The listing builds one solid part. Answer for the finished solid, in the listing's coordinates (mm). A direction names the side the tool comes from. Give positions to 0.01 mm unless a question says otherwise; leave off trailing zeros. Write each loop counter-clockwise with the first axis right and the second up, starting at its lowest first coordinate (ties: lowest second). Pieces come first, ordered by that corner, then holes. Notation, with made-up numbers: (-23, -7.75) - (0, -7.75) arc R21 cw to (0, -1.75) - close; hole circle Ø1 at (59.5, 39.25). An arc over 180 degrees is marked (long way). Answer as CSV lines item,"result". Start each with the question number.
(1) For faces 4 (the face through (184.08, -0.99, 126.32)), 5 (the face through (182.017, -1.479, 125.126)), determine the directions among +Z, -Z, +X, -X, +Y, -Y from which every point of the face is accessible in a straight line to the end or side of a thin tool.
(2) Find section A-A (x = 184.15). Write down the section's boundary in (y, z), then the cut area to 3 significant figures.
(3) Find section B-B (y = -0.75). Write down the section's boundary in (x, z), then the cut area to 3 significant figures.
(4) For a pull along X with two mould halves and no side action, classify faces 1 (the face through (183.37, -6.85, 124.21)), 2 (the face through (183.464, -1, 125)), 3 (the face through (183, -3, 126)) as pulls with the +X half, pulls with the -X half, needs draft (parallel to the pull), parting line crosses it, or undercut.
(5) Straight lines are drawn through the part: probe 1 along Y at (x, z) = (182.45, 125.45); probe 2 along Y at (x, z) = (183.5, 125.2); probe 3 along X at (y, z) = (-9, 125.35). For each, find the intervals that lie inside material, in ascending order.
(6) Find section C-C (z = 124.4). Write down the section's boundary in (x, y), then the cut area to 3 significant figures.
(7) Each of these flat-tipped pins is pushed along its axis until it touches: pin 1 Ø2 at (y, z) = (-5, 124) entering from -X; pin 2 Ø1 at (x, z) = (183, 127) entering from -Y. Where does it stop, or does it pass through?
(8) Find section D-D (y = -9.25). Write down the section's boundary in (x, z), then the cut area to 3 significant figures.
from build123d import *

# Parameters (mm, degrees)
SKETCH1_R           = 2.7
BOSS_EXTRUDE1_DEPTH = 3
SKETCH2_R           = 1.696293742
BOSS_EXTRUDE2_DEPTH = 7.8
CUT_EXTRUDE1_DEPTH  = 2


with BuildPart() as part:
    # Sketch1 → Boss-Extrude1 (new body)
    with BuildSketch(Plane(origin=(0, 0, 0), x_dir=(1, 0, 0), z_dir=(0, 1, 0))):
        with Locations((184.714490272, -125.24429514)):
            Circle(SKETCH1_R)
    extrude(amount=-BOSS_EXTRUDE1_DEPTH)

    # Sketch2 → Boss-Extrude2 (add)
    with BuildSketch(Plane.XZ.offset(3)):
        with Locations((184.714490272, 125.24429514)):
            Circle(SKETCH2_R)
    extrude(amount=BOSS_EXTRUDE2_DEPTH)

    # Sketch3 → Cut-Extrude1 (cut)
    with BuildSketch(Plane(origin=(0, 0, 0), x_dir=(1, 0, 0), z_dir=(0, 1, 0))):
        Polygon((184.714490272, -123.800919467), (183.464490272, -124.522607304), (183.464490272, -125.965982977), (184.714490272, -126.687670813), (185.964490272, -125.965982977), (185.964490272, -124.522607304), align=None)
    extrude(amount=-CUT_EXTRUDE1_DEPTH, mode=Mode.SUBTRACT)


solid = part.part
Result set:
1,face 4,"+Y"
1,face 5,"+Y, -Y"
2,outline,"(-10.8, 123.64) - (-3, 123.64) - (-3, 122.6) - (0, 122.6) - (0, 124.13) - (-2, 124.13) - (-2, 126.36) - (0, 126.36) - (0, 127.88) - (-3, 127.88) - (-3, 126.84) - (-10.8, 126.84) - close"
2,area,"36.3 mm^2"
3,outline,"circle Ø5.4 at (184.71, 125.24); hole (183.46, 124.52) - (184.71, 123.8) - (185.96, 124.52) - (185.96, 125.97) - (184.71, 126.69) - (183.46, 125.97) - close"
3,area,"17.5 mm^2"
4,face 1,"parting line crosses it"
4,face 2,"undercut"
4,face 3,"needs draft"
5,probe 1,"-3 to 0"
5,probe 2,"-10.8 to -2"
5,probe 3,"183.02 to 186.41"
6,outline,"(182.15, -3) - (183.24, -3) - (183.24, -10.8) - (186.19, -10.8) - (186.19, -3) - (187.28, -3) - (187.28, 0) - (185.75, 0) - (185.75, -2) - (183.68, -2) - (183.68, 0) - (182.15, 0) - close"
6,area,"34.2 mm^2"
7,pin 1,"x = 183.04"
7,pin 2,"y = -3"
8,outline,"circle Ø3.39 at (184.71, 125.24)"
8,area,"9.04 mm^2"
